Geometry check sheet. Reference: the model listing, model coordinates, mm. A direction names the side the tool comes from. Round coordinates to 2 decimals unless told otherwise and drop trailing zeros. Loops run counter-clockwise (first coordinate to the right, second up) from the corner with the lowest first, then second, coordinate; pieces in that order, holes last. Notation, with made-up numbers: M -16,14.5 L 17,14.5 A22 cw 17,24.5 Z; hole C -11.75,-29 d3. An arc over 180 degrees is marked long. Answer in a Markdown table with one row per item. Add a question column.
```python
from build123d import *

# Parameters (mm, degrees)
SKETCH1_R           = 2.5
SKETCH1_R_2         = 1
BOSS_EXTRUDE1_DEPTH = 1.5


with BuildPart() as part:
    # Sketch1 → Boss-Extrude1 (new body)
    with BuildSketch(Plane(origin=(0, 0, 0), x_dir=(1, 0, 0), z_dir=(0, 1, 0))):
        Polygon((-7.9, 71.58), (-46.39309335, 71.58), (-46.39309335, 51.58), (-21.023384775, 2), (0, 2), (0, 51.58), (-7.9, 51.58), align=None)
        with Locations(Location((-17.9, 61.58, 0), (0, 0, 270))):
            Circle(SKETCH1_R, mode=Mode.SUBTRACT)
        with Locations(Location((-39.39309335, 61.58, 0), (0, 0, 270))):
            Circle(SKETCH1_R, mode=Mode.SUBTRACT)
        with Locations(Location((-5, 7.14, 0), (0, 0, 270))):
            Circle(SKETCH1_R_2, mode=Mode.SUBTRACT)
        with Locations(Location((-15, 7.14, 0), (0, 0, 270))):
            Circle(SKETCH1_R_2, mode=Mode.SUBTRACT)
    extrude(amount=BOSS_EXTRUDE1_DEPTH)


solid = part.part
```
1) Cross-section at A-A, the plane x = -5. Record the boundary of the cut face in (y, z), plus the area to 3 significant figures.
2) Cross-section at B-B, the plane z = -61.58. Record the boundary of the cut face in (x, y), plus the area to 3 significant figures.
3) Go/stop test with a flat-tipped pin: pin 1 (0.8 mm diameter, centred on y = 1, z = -57, fed in from +X). Record where the tip stops, or that it passes through.
4) Cross-section at C-C, the plane y = 0.95. Record the boundary of the cut face in (x, z).
5) Set-up check for faces 1 (the flat face through (0, 1, -26)), 2 (the flat face through (-4, 1, -51.58)): record each of +Z, -Z, +X, -X, +Y, -Y from which the full face is reachable in a straight line by a thin tool's end or side.
6) Thickness scan on L1, parallel to X at y = 1, z = -61.58; L2, parallel to X at y = 1.25, z = -7.14; L3, parallel to Z at x = -39, y = 1.2. Record the ranges inside material, lowest first. Write a range as [from, to].
7) Cross-section at D-D, the plane x = -17.9. Record the boundary of the cut face in (y, z), plus the area to 3 significant figures.
8) Draft check along X on faces 3 (the flat face through (-33.886, 0.74, -27.137)), 4 (the cylindrical face through (-17.149, 0.74, -59.195)), 5 (the flat face through (-18, 0, -37)). Enter one of: +X half, -X half, draft (parallel to the pull), parting line (faces both ways), or undercut.
Worked answers:
| question | item | result |
|---|---|---|
| 1 | outline | M 0,-51.58 L 1.5,-51.58 L 1.5,-8.14 L 0,-8.14 Z; M 0,-6.14 L 1.5,-6.14 L 1.5,-2 L 0,-2 Z |
| 1 | area | 71.4 mm2 |
| 2 | outline | M -46.39,0 L -41.89,0 L -41.89,1.5 L -46.39,1.5 Z; M -36.89,0 L -20.4,0 L -20.4,1.5 L -36.89,1.5 Z; M -15.4,0 L -7.9,0 L -7.9,1.5 L -15.4,1.5 Z |
| 2 | area | 42.7 mm2 |
| 3 | pin 1 | stops at x = -7.9 |
| 4 | outline | M -46.39,-71.58 L -7.9,-71.58 L -7.9,-51.58 L 0,-51.58 L 0,-2 L -21.02,-2 L -46.39,-51.58 Z; hole C -39.39,-61.58 d5; hole C -17.9,-61.58 d5; hole C -15,-7.14 d2; hole C -5,-7.14 d2 |
| 5 | face 1 | +Z, -Z, +X, +Y, -Y |
| 5 | face 2 | -Z, +X, +Y, -Y |
| 6 | L1 | x = [-46.39, -41.89], [-36.89, -20.4], [-15.4, -7.9] |
| 6 | L2 | x = [-23.65, -16], [-14, -6], [-4, 0] |
| 6 | L3 | z = [-71.58, -64.05], [-59.11, -37.13] |
| 7 | outline | M 0,-71.58 L 1.5,-71.58 L 1.5,-64.08 L 0,-64.08 Z; M 0,-59.08 L 1.5,-59.08 L 1.5,-2 L 0,-2 Z |
| 7 | area | 96.9 mm2 |
| 8 | face 3 | -X half |
| 8 | face 4 | undercut |
| 8 | face 5 | draft |
